Could you check a few things on this model? Use its own coordinates, in mm. Give positions to 0.01 mm unless a question says otherwise; leave off trailing zeros. Loops run counter-clockwise (first coordinate to the right, second up) from the corner with the lowest first, then second, coordinate; pieces in that order, holes last.
1. I need wall thicknesses on line 1 along Y through (x, z) = (150, 0.9); line 2 along Y through (x, z) = (-85.4, 2.5); line 3 along Y through (x, z) = (10, 2.3). Which ranges of each line are inside material? Lowest first, please.
2. Imagine slicing it at A-A (x = -85.4). List the corners of the cut face in (y, z) for me, plus the area to 3 significant figures.
3. Thinking about a two-plate mould opening in X: for faces 1 (the flat face through (-2, 1, 0)), 2 (the cylindrical face through (-88.04, -87.58, 1.73)), which applies, +X half, -X half, draft (parallel to the pull), parting line (faces both ways), or undercut?
Autodesk Inventor part; units mm, degrees
ref_plane "YZ Plane" through (0, 0, 0) normal (1, 0, 0) x (0, 1, 0)
ref_plane "XZ Plane" through (0, 0, 0) normal (0, 1, 0) x (-1, 0, 0)
ref_plane "XY Plane" through (0, 0, 0) normal (0, 0, 1) x (1, 0, 0)
sketch "Sketch1" plane through (0, 0, 0) normal (0, 0, 1) x (1, 0, 0)
  line L0 (-160, 100) -> (160, 100)
  line L1 (160, 100) -> (160, -100)
  line L2 (160, -100) -> (-160, -100)
  line L3 (-160, -100) -> (-160, 100)
  point P0 (0, 0)
  dimension "d0" = 320
  dimension "d1" = 200
  dimension "d2" = 160
  dimension "d3" = 100
extrude "Extrusion1" add sketch "Sketch1" along normal blind 3.4163
sketch "Sketch2" plane through (0, 0, 3.4163) normal (0, 0, 1) x (1, 0, 0)
  line L0 (160, 100) -> (-160, 100)
  line L1 (-160, 100) -> (-160, -100)
  line L2 (-160, -100) -> (160, -100)
  line L3 (160, -100) -> (160, 100)
  circle A0 centre (-150, -90) radius 2.75
  circle A1 centre (-150, 90) radius 2.75
  circle A2 centre (-85.4, 90) radius 3.58
  circle A3 centre (-85.4, -90) radius 3.58
  circle A4 centre (85.4, 90) radius 3.58
  circle A5 centre (150, 90) radius 2.75
  circle A6 centre (85.4, -90) radius 3.58
  circle A7 centre (150, -90) radius 2.75
  point P0 (0, 0)
  dimension "d6" = 5.5
  dimension "d7" = 5.5
  dimension "d8" = 7.16
  dimension "d9" = 7.16
  dimension "d10" = 7.16
  dimension "d11" = 5.5
  dimension "d12" = 7.16
  dimension "d13" = 5.5
  dimension "d14" = 10
  dimension "d15" = 10
  dimension "d16" = 64.6
  dimension "d17" = 10
  dimension "d18" = 64.6
  dimension "d19" = 10
  dimension "d20" = 10
  dimension "d21" = 10
  dimension "d22" = 10
  dimension "d23" = 10
  dimension "d24" = 10
  dimension "d25" = 10
  dimension "d26" = 10
  dimension "d27" = 64.6
  dimension "d28" = 64.6
  dimension "d29" = 10
extrude "Extrusion2" cut sketch "Sketch2" against normal through all contours A0 | A1 | A2 | A3 | A4 | A5 | A6 | A7
fillet "Fillet1" radius 5 4 edges at (-160, -100, 1.7082) (-160, 100, 1.7082) (160, 100, 1.7082) (160, -100, 1.7082)
sketch "Sketch3" plane through (0, 0, 0) normal (0, 0, -1) x (-1, 0, 0)
  circle A0 centre (-10, 0) radius 2.067
  circle A1 centre (10, 0) radius 2.067
  circle A2 centre (-10, 0) radius 2.75
  circle A3 centre (10, 0) radius 2.75
  point P0 (0, 0)
  dimension "d33" = 5.5
  dimension "d34" = 5.5
extrude "Extrusion3" cut sketch "Sketch3" against normal through all contours A0 | A1 | A2 | A3
sketch "Sketch4" plane through (0, 0, 0) normal (0, 0, -1) x (-1, 0, 0)
  line L0 (-155, -100) -> (155, -100)
  line L1 (-160, 95) -> (-160, -95)
  circle A0 centre (-120, -90) radius 2.75
  point P0 (0, 0)
  dimension "d37" = 5.5
  dimension "d38" = 40
  dimension "d39" = 10
extrude "Extrusion4" cut sketch "Sketch4" against normal through all
pattern_linear "Rectangular Pattern1" count 2 spacing 240 along (-1, 0, 0) count 2 spacing 180 along (0, 1, 0) of "Extrusion4"
properties part number "y-carriage" material "Steel, Mild"
Derived:
1. line 1: y = -100 to -92.75, -87.25 to 87.25, 92.75 to 100
1. line 2: y = -100 to -93.58, -86.42 to 86.42, 93.58 to 100
1. line 3: y = -100 to -2.75, 2.75 to 100
2. outline: (-100, 0) - (-93.58, 0) - (-93.58, 3.42) - (-100, 3.42) - close; (-86.42, 0) - (86.42, 0) - (86.42, 3.42) - (-86.42, 3.42) - close; (93.58, 0) - (100, 0) - (100, 3.42) - (93.58, 3.42) - close
2. area: 634 mm2
3. face 1: draft
3. face 2: undercut
